Could you check a few things on this drawing? It's one solid part, dimensions in mm from its lowest x, y, z. A direction names the side the tool comes from. Coordinates: 2 decimals unless noted, no trailing zeros. Loops run counter-clockwise (first coordinate to the right, second up) from the corner with the lowest first, then second, coordinate; pieces in that order, holes last. Notation, with made-up numbers: M 18,17.25 L 29,17.25 A15 ccw 29,28.25 Z; hole C 37.25,9.25 d11. An arc over 180 degrees is marked long. Use one line per item in the form item = value. Start each with the question number.
(1) Imagine slicing it at B-B, the plane y = 4.75. Please give me the cut outline in (x, z).
(2) On a 3-axis mill with a long thin cutter (end or side, diameter ignored), from which of +Z, -Z, +X, -X, +Y, -Y can I reach the whole of each face in a straight line? I mean the marked faces 5 and 6. Say none if no direction works.
(3) Please list where these lines run through material, in increasing order: L1, parallel to Z at x = 11, y = 4.65; L2, parallel to Y at x = 12.5, z = 10; L3, parallel to Z at x = 11, y = 1.15.
(4) Imagine slicing it at A-A, the plane x = 11. State how many separate pieces and enclosed holes the cut face has, and give its area (3 significant figures).
(5) Thinking about a two-plate mould opening in Z: for the marked faces 1, 2, 3 and 4, which applies, +Z half, -Z half, draft (parallel to the pull), parting line (faces both ways), or undercut?
(6) Will these pins go through, and if not, where does the flat tip stop? P1, Ø3, axis at y = 2.5, z = 10, coming from the +X side; P2, Ø4, axis at x = 4, z = 2.5, coming from the -Y side; P3, Ø2, axis at y = 3.5, z = 12.5, coming from the +X side.
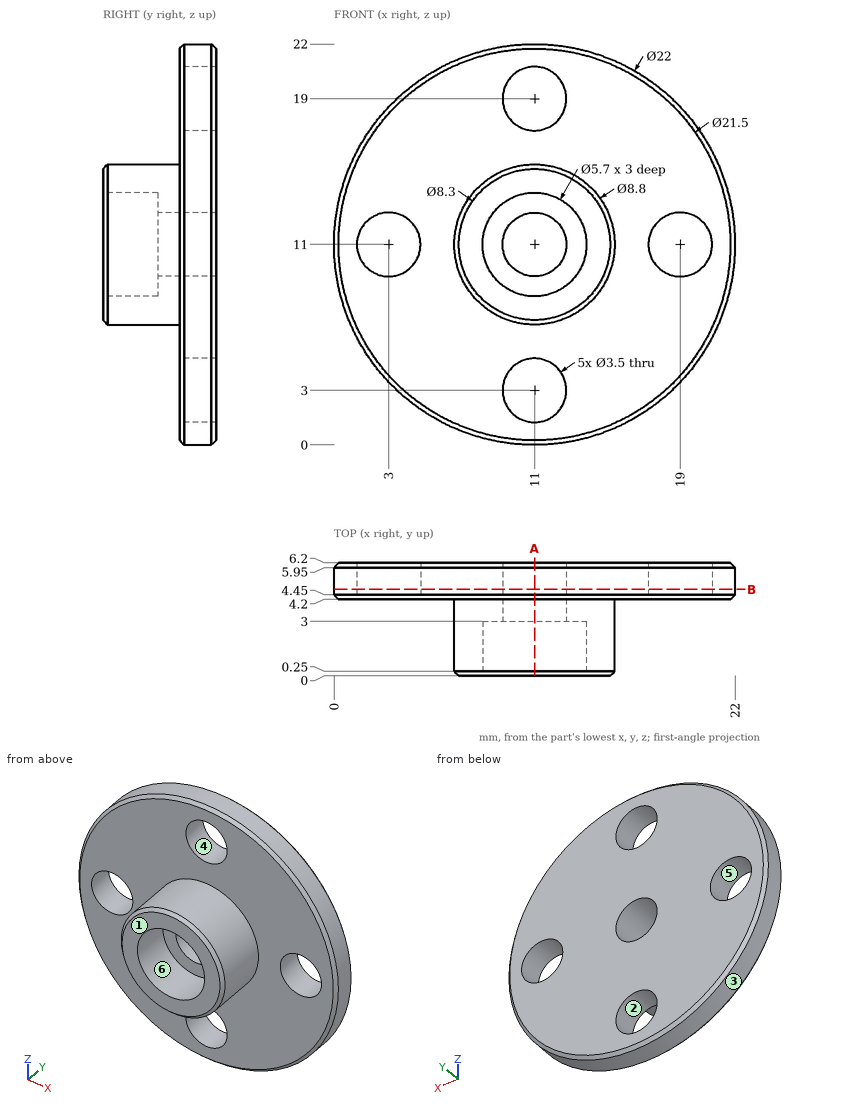
Answer:
q1.outline = C 11,11 d22; hole C 3,11 d3.5; hole C 11,3 d3.5; hole C 11,11 d3.5; hole C 11,19 d3.5; hole C 19,11 d3.5
q2.face_5 = +Y, -Y
q2.face_6 = -Y
q3.L1 = 0 to 1.25, 4.75 to 9.25, 12.75 to 17.25, 20.75 to 22
q3.L2 = 3 to 6.2
q3.L3 = 6.6 to 8.15, 13.85 to 15.4
q4.separate_pieces = 4
q4.enclosed_holes = 0
q4.area = 38.5 mm²
q5.face_1 = draft
q5.face_2 = undercut
q5.face_3 = parting line
q5.face_4 = undercut
q6.P1 = 15.4
q6.P2 = 4.2
q6.P3 = 21.94
